Build history of the part. All positions in model axes, mm. Round coordinates to 2 decimals unless told otherwise and drop trailing zeros. Order: outer loops, then holes, each group sorted by start corner. A loop starts at its lowest first (then second) coordinate and runs counter-clockwise, first axis right, second up. Notation, with made-up numbers: (51, -24.75) -> (57, -24.75) arc R9 cw to (57, -11.75) -> close; hole circle Ø6 at (35.5, 73.25). An arc over 180 degrees is marked (long way). Use a Markdown table: item, result. Add a question column.
Item 1: Probe L1, parallel to Z at x = 1, y = 18; L2, parallel to Y at x = 1, z = -7.5; L3, parallel to Z at x = 0.6, y = 14.5. List the from-to ranges inside material, lowest first.
Item 2: Slice it at C-C, the plane z = -13. Give the cut face in (x, y).
Item 3: Slice it at B-B, the plane x = 1.3. Give the cut face in (y, z).
Item 4: Slice it at A-A, the plane y = 23. Give the cut face in (x, z) (3 decimals).
Item 5: Slice it at D-D, the plane y = 30. Give the cut face in (x, z) (3 decimals), plus the area to 3 significant figures.
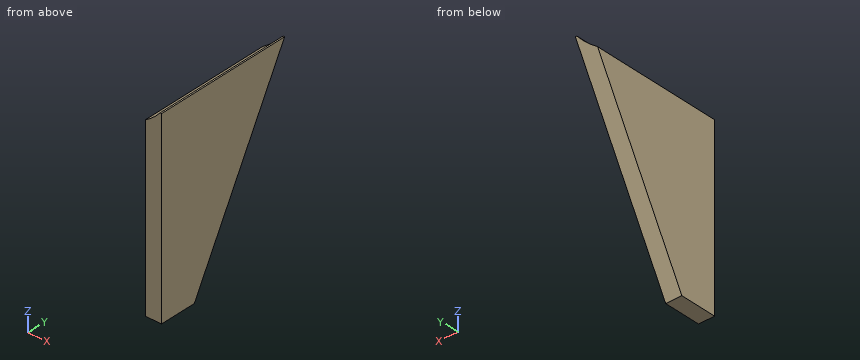
from build123d import *

# Parameters (mm, degrees)
BOSS_EXTRUDE1_DEPTH = 3.77
FILLET1_R           = 0.2
CAVITY1_DEPTH       = 32.53
CUT_EXTRUDE1_DEPTH  = 10


# Read off the part's stored shape, not the designer's step: Cavity1
with BuildPart() as part:
    # Sketch1 → Boss-Extrude1 (new body)
    with BuildSketch(Plane(origin=(0, 0, 0), x_dir=(0, 0, -1), z_dir=(1, 0, 0))):
        Polygon((0, 0), (60, 0), (0, 32.53), align=None)
    extrude(amount=BOSS_EXTRUDE1_DEPTH)

    # Fillet1
    fillet1_edges = [part.edges().sort_by_distance(p)[0] for p in [
        (1.885, 0, -60),
    ]]
    fillet(fillet1_edges, radius=FILLET1_R)

    # Cavity1 outline → Cavity1 (cut)
    with BuildSketch(Plane(origin=(0, 0, 0), x_dir=(1, 0, 0), z_dir=(0, 1, 0))):
        with BuildLine():
            Line((0, 0), (3.434066763, 0))
            ThreePointArc((3.434066763, 0), (1.851918424, 1.627143202), (0, 2.939083185))
            Line((0, 2.939083185), (0, 0))
        make_face()
    extrude(amount=CAVITY1_DEPTH, mode=Mode.SUBTRACT)

    # Sketch2 → Cut-Extrude1 (cut)
    with BuildSketch(Plane.ZY):
        Polygon((-44.024699242, 0), (-44.024699242, 8.661275561), (-59.306815437, 0.375821564), (-59.211490846, 0), align=None)
    extrude(amount=-CUT_EXTRUDE1_DEPTH, mode=Mode.SUBTRACT)


with BuildPart() as body_2:
    # of the pieces the cut leaves, the one that is kept (cut_extrude1_keep)
    add(part.part.solids().sort_by_distance((0, 0, -2.939083185))[0])


solid = body_2.part
Check sheet entries:
| question | item | result |
|---|---|---|
| 1 | L1 | -26.8 to -2.29 |
| 1 | L2 | 0 to 28.46 |
| 1 | L3 | -33.26 to -2.57 |
| 2 | outline | (0, 0) -> (3.77, 0) -> (3.77, 25.48) -> (0, 25.48) -> close |
| 3 | outline | (0, -44.02) -> (8.66, -44.02) -> (31.41, -2.07) -> (0, -2.07) -> close |
| 4 | outline | (0, -17.578) -> (3.77, -17.578) -> (3.77, 0) -> (3.434, 0) arc R12.415 cw to (0, -2.939) -> close |
| 5 | outline | (0, -4.666) -> (3.77, -4.666) -> (3.77, 0) -> (3.434, 0) arc R12.415 cw to (0, -2.939) -> close |
| 5 | area | 11.9 mm2 |
